Could you check a few things on this model? Use its own coordinates, in mm. A direction names the side the tool comes from. Round coordinates to 2 decimals unless told otherwise and drop trailing zeros. Write each loop counter-clockwise with the first axis right and the second up, starting at its lowest first coordinate (ties: lowest second). Pieces come first, ordered by that corner, then holes. Notation, with made-up numbers: (74.25, 52) -> (107.25, 52) arc R11 cw to (107.25, 64) -> close; hole circle Ø5 at (-4.75, 59). An arc over 180 degrees is marked (long way). Return JSON: item names as keys, results as strings.
from build123d import *

# Parameters (mm, degrees)
F0_W     = 8
F0_H     = 1.6
F2_DEPTH = 1.4


with BuildPart() as f2:
    # F0 (on Top) → F2 (new body)
    with BuildSketch(Plane.XY):
        with Locations((-9, -20.3)):
            Rectangle(F0_W, F0_H)
        with Locations((-9, 20.3)):
            Rectangle(F0_W, F0_H)
        Polygon((-13, 19.5), (-18.4, 19.5), (-18.4, -19.5), (-13, -19.5), (-5, -19.5), (5, -19.5), (13, -19.5), (18.4, -19.5), (18.4, 19.5), (13, 19.5), (5, 19.5), (-5, 19.5), align=None)
        with Locations((9, 20.3)):
            Rectangle(F0_W, F0_H)
        with Locations((9, -20.3)):
            Rectangle(F0_W, F0_H)
    extrude(amount=F2_DEPTH)


solid = f2.part
1) Will these pins go through, and if not, where does the flat tip stop? pin 1 Ø0.7 at (y, z) = (20.5, 1) entering from -X; pin 2 Ø0.7 at (x, z) = (-2, 0.5) entering from +Y.
Return value:
{"pin 1": "x = -13", "pin 2": "y = 19.5"}
2) For faces 1 (the face through (16, 19.5, 1)), 2 (the face through (-13, -20, 1)), 3 (the face through (0, -19.5, 1)), 4 (the face through (5, 20, 1)), 5 (the face through (-16, 19.5, 1)), which set-ups out of +Z, -Z, +X, -X, +Y, -Y let a thin tool reach every point of the face, with its end or its side?
Return value:
{"face 1": "+Z, -Z, +X, +Y", "face 2": "+Z, -Z, -X, -Y", "face 3": "+Z, -Z, -Y", "face 4": "+Z, -Z, +Y", "face 5": "+Z, -Z, -X, +Y"}
3) I want a section at B-B, the plane x = 3. Please give me the cut outline in (y, z), and give its area (3 significant figures).
Return value:
{"outline": "(-19.5, 0) -> (19.5, 0) -> (19.5, 1.4) -> (-19.5, 1.4) -> close", "area": "54.6 mm²"}
4) Thinking about a two-plate mould opening in X: for faces 6 (the face through (0, 0, 1.4)), 7 (the face through (13, 20, 1)), 8 (the face through (0, 19.5, 1)), 9 (the face through (-13, 20, 1)), which applies, pulls with the +X half, pulls with the -X half, needs draft (parallel to the pull), parting line crosses it, or undercut?
Return value:
{"face 6": "needs draft", "face 7": "pulls with the +X half", "face 8": "undercut", "face 9": "pulls with the -X half"}
5) I want a section at A-A, the plane z = 0.25. Please give me the cut outline in (x, y).
Return value:
{"outline": "(-18.4, -19.5) -> (-13, -19.5) -> (-13, -21.1) -> (-5, -21.1) -> (-5, -19.5) -> (5, -19.5) -> (5, -21.1) -> (13, -21.1) -> (13, -19.5) -> (18.4, -19.5) -> (18.4, 19.5) -> (13, 19.5) -> (13, 21.1) -> (5, 21.1) -> (5, 19.5) -> (-5, 19.5) -> (-5, 21.1) -> (-13, 21.1) -> (-13, 19.5) -> (-18.4, 19.5) -> close"}
6) If I drill on probe 1 along Y at (x, z) = (-4.5, 0.2), over which ranges is the centre line in solid material (lowest first)? Write a range as [from, to].
Return value:
{"probe 1": "[-19.5, 19.5]"}
